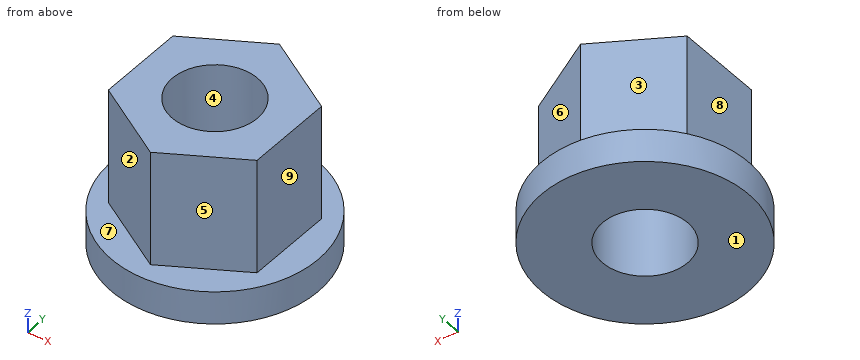
from build123d import *

# Parameters (mm, degrees)
F0_R     = 12.5
F1_DEPTH = 4
F3_DEPTH = 14
F5_D     = 10.3


with BuildPart() as f1:
    # F0 (on Top) → F1 (new body)
    with BuildSketch(Plane.XY):
        Circle(F0_R)
    extrude(amount=-F1_DEPTH)

    # F2 (on face) → F3 (join)
    with BuildSketch(Plane.XY):
        Polygon((9, -5.1961524227), (9, 5.1961524227), (0, 10.3923048454), (-9, 5.1961524227), (-9, -5.1961524227), (0, -10.3923048454), align=None)
    extrude(amount=F3_DEPTH)

    # F5 (through all)
    with Locations(Plane(origin=(0, 0, -4), x_dir=(1, 0, 0), z_dir=(0, 0, -1))):
        with Locations((0, 0)):
            Hole(F5_D / 2)


solid = f1.part
Input: part model. Units: mm. Frame: model coordinates. Face numbers are marked on the shaded views. A direction names the side the tool comes from. Coordinates: 2 decimals unless noted, no trailing zeros. Loops run counter-clockwise (first coordinate to the right, second up) from the corner with the lowest first, then second, coordinate; pieces in that order, holes last. Notation, with made-up numbers: (-32, 79) -> (-6, 79) arc R15 cw to (-6, 105) -> close; hole circle Ø10 at (-32.5, 38.5). An arc over 180 degrees is marked (long way). Write item = value, one per line. Start each with the question number.
Item 1: Reachability of the marked faces 5, 6, 7, 8 and 9 from +Z, -Z, +X, -X, +Y, -Y: full face, straight path, thin tool, end or side. Return the list, or none.
Item 2: First-contact query: P1, Ø6, axis at x = -2, y = 1.5, coming from the -Z side; P2, Ø2, axis at x = -4, z = 0, coming from the -Y side; P3, Ø5, axis at y = -7.5, z = 11.5, coming from the -X side; P4, Ø8, axis at x = -7, z = 4.5, coming from the +Y side. Flat tips, straight axial feed; report the tip coordinate or a pass-through.
Item 3: Mould query, pull axis Y, two halves, no side actions, for the marked faces 1, 2, 3 and 4. Classes: pulls with the +Y half, pulls with the -Y half, needs draft (parallel to the pull), parting line crosses it, or undercut.
Item 4: Cut plane D-D, the plane y = -10. Return loops of the section in (x, z), plus the area to 3 significant figures.
Item 5: Cut plane B-B, the plane y = 0. Return loops of the section in (x, z), plus the area to 3 significant figures.
Item 6: Cut plane C-C, the plane x = -4.5. Return loops of the section in (y, z), plus the area to 3 significant figures.
Item 7: Material intervals for line 1 (X direction, y = -2, z = -1.75); line 2 (Z direction, x = -4.25, y = -8.75); line 3 (Y direction, x = 2.5, z = 4.5), sorted ascending.
Item 8: Cut plane A-A, the plane z = 11. Return loops of the section in (x, y), plus the area to 3 significant figures.
Ans:
q1.face_5 = +Z, +X, -Y
q1.face_6 = +Z, +X, +Y
q1.face_7 = +Z
q1.face_8 = +Z, -X, +Y, -Y
q1.face_9 = +Z, +X, +Y, -Y
q2.P1 = -4
q2.P2 = -12.13
q2.P3 = -9
q2.P4 = 8.66
q3.face_1 = needs draft
q3.face_2 = pulls with the -Y half
q3.face_3 = pulls with the +Y half
q3.face_4 = undercut
q4.outline = (-7.5, -4) -> (7.5, -4) -> (7.5, 0) -> (0.68, 0) -> (0.68, 14) -> (-0.68, 14) -> (-0.68, 0) -> (-7.5, 0) -> close
q4.area = 79.0 mm²
q5.outline = (-12.5, -4) -> (-5.15, -4) -> (-5.15, 14) -> (-9, 14) -> (-9, 0) -> (-12.5, 0) -> close; (5.15, -4) -> (12.5, -4) -> (12.5, 0) -> (9, 0) -> (9, 14) -> (5.15, 14) -> close
q5.area = 167 mm²
q6.outline = (-11.66, -4) -> (-2.5, -4) -> (-2.5, 14) -> (-7.79, 14) -> (-7.79, 0) -> (-11.66, 0) -> close; (2.5, -4) -> (11.66, -4) -> (11.66, 0) -> (7.79, 0) -> (7.79, 14) -> (2.5, 14) -> close
q6.area = 221 mm²
q7.line_1 = -12.34 to -4.75, 4.75 to 12.34
q7.line_2 = -4 to 0
q7.line_3 = -8.95 to -4.5, 4.5 to 8.95
q8.outline = (-9, -5.2) -> (0, -10.39) -> (9, -5.2) -> (9, 5.2) -> (0, 10.39) -> (-9, 5.2) -> close; hole circle Ø10.3 at (0, 0)
q8.area = 197 mm²
